Work out the finished part from the listing and answer in its coordinate system (mm). Coordinates: 2 decimals unless noted, no trailing zeros. Loops run counter-clockwise (first coordinate to the right, second up) from the corner with the lowest first, then second, coordinate; pieces in that order, holes last. Notation, with made-up numbers: (80.5, -39) - (128.5, -39) arc R29 ccw to (128.5, -11) - close; hole circle Ø7 at (5.5, 1.5). An arc over 180 degrees is marked (long way). Write each question's results on one line, items separated by ' | '. Start each with the question number.
Item 1: For a pull along Y with two mould halves and no side action, classify faces 1 (the face through (-80.22, -125.83, -2.13)), 2 (the face through (-101, 112, 152.4)), 3 (the face through (19.839, -151.103, 2.134)) as +Y half, -Y half, draft (parallel to the pull), parting line (faces both ways), or undercut.
Item 2: Section B-B, the plane x = 93 is taken. Write down the section's boundary in (y, z).
Item 3: Section A-A, the plane y = 0 is taken. Write down the section's boundary in (x, z) (3 decimals).
Item 4: Section C-C, the plane z = 51.5 is taken. Write down the section's boundary in (x, y) (3 decimals).
Item 5: Consider probe 1 along Y at (x, z) = (0, 75) (3 decimals); probe 2 along Y at (x, z) = (0, -57) (3 decimals); probe 3 along X at (y, z) = (-79, 74.5). Determine where each line is inside the solid, lowest interval first. Write a range as [from, to].
Item 6: Section D-D, the plane x = 0 is taken. Count the separate pieces of the cut face and the enclosed holes in it, plus the area to 3 significant figures.
Item 7: Each of these flat-tipped pins is pushed along its axis until it touches: pin 1 Ø1.5 at (x, z) = (25.5, -77) entering from +Y; pin 2 Ø2 at (y, z) = (44.5, -21) entering from +X; pin 3 Ø12 at (x, z) = (-88.5, 27) entering from +Y. Where does it stop, or does it pass through?
from build123d import *

# Parameters (mm, degrees)
SKETCH3_R                                = 152.4
SKETCH3_R_2                              = 149.225
BOSS_EXTRUDE1_DEPTH                      = 152.4
F_1_0MM_DOWEL_HOLE1_REACH                = 394.408
F_1_0MM_DOWEL_HOLE1_BORE_R               = 38.5
F_1_2_0_5_DIAMETER_HOLE1_REACH           = 394.606
F_1_2_0_5_DIAMETER_HOLE1_BORE_R          = 6.35
F_1_2_0_5_DIAMETER_HOLE1_ON_FACE_2_REACH = 387.1
F_1_2_0_5_DIAMETER_HOLE1_BORE_2_R        = 6.35


with BuildPart() as part:
    # Sketch3 → Boss-Extrude1 (new, symmetric)
    with BuildSketch(Plane.XY):
        with Locations(Location((0, 0, 0), (0, 0, 180))):
            Circle(SKETCH3_R)
        with Locations(Location((0, 0, 0), (0, 0, 180))):
            Circle(SKETCH3_R_2, mode=Mode.SUBTRACT)
    extrude(amount=BOSS_EXTRUDE1_DEPTH, both=True)

    # Ø1.0mm Dowel Hole1 bore (on position points) → Ø1.0mm Dowel Hole1 (cut, up to next)
    with BuildSketch(Plane(origin=(-1.237560308, 152.394975129, -41.195571985), x_dir=(0.999967028404, 0.008120474463, 0), z_dir=(-0.008120474463, 0.999967028404, 0)), mode=Mode.PRIVATE) as f_1_0mm_dowel_hole1_sk1:
        Circle(F_1_0MM_DOWEL_HOLE1_BORE_R)
    f_1_0mm_dowel_hole1_tool1 = extrude(f_1_0mm_dowel_hole1_sk1.sketch, amount=-F_1_0MM_DOWEL_HOLE1_REACH, mode=Mode.PRIVATE) & part.part
    add(f_1_0mm_dowel_hole1_tool1.solids().sort_by_distance((-1.23756, 152.394975, -41.195572))[0], mode=Mode.SUBTRACT)

    # 1/2 (0.5) Diameter Hole1 bore (on position points) → 1/2 (0.5) Diameter Hole1 (cut, up to next)
    with BuildSketch(Plane(origin=(-0.547224497, -152.399017534, -42.136286286), x_dir=(-0.999993553373, 0.003590711924, 0), z_dir=(-0.003590711924, -0.999993553373, 0)), mode=Mode.PRIVATE) as f_1_2_0_5_diameter_hole1_sk1:
        Circle(F_1_2_0_5_DIAMETER_HOLE1_BORE_R)
    f_1_2_0_5_diameter_hole1_tool1 = extrude(f_1_2_0_5_diameter_hole1_sk1.sketch, amount=-F_1_2_0_5_DIAMETER_HOLE1_REACH, mode=Mode.PRIVATE) & part.part
    add(f_1_2_0_5_diameter_hole1_tool1.solids().sort_by_distance((-0.547224, -152.399018, -42.136286))[0], mode=Mode.SUBTRACT)

    # 1/2 (0.5) Diameter Hole1 bore 2 (on position points) → 1/2 (0.5) Diameter Hole1 on face 2 (cut, up to next)
    with BuildSketch(Plane(origin=(0.182408166, -152.399890837, 26.814000364), x_dir=(-0.999999283595, -0.001197000339, 0), z_dir=(0.001197000339, -0.999999283595, 0)), mode=Mode.PRIVATE) as f_1_2_0_5_diameter_hole1_on_face_2_sk1:
        Circle(F_1_2_0_5_DIAMETER_HOLE1_BORE_2_R)
    f_1_2_0_5_diameter_hole1_on_face_2_tool1 = extrude(f_1_2_0_5_diameter_hole1_on_face_2_sk1.sketch, amount=-F_1_2_0_5_DIAMETER_HOLE1_ON_FACE_2_REACH, mode=Mode.PRIVATE) & part.part
    add(f_1_2_0_5_diameter_hole1_on_face_2_tool1.solids().sort_by_distance((0.182408, -152.399891, 26.814))[0], mode=Mode.SUBTRACT)


solid = part.part
Answer key:
1) face 1: undercut | face 2: draft | face 3: parting line
2) outline: (-120.73, -152.4) - (-116.7, -152.4) - (-116.7, 152.4) - (-120.73, 152.4) - close; (116.7, -152.4) - (120.73, -152.4) - (120.73, 152.4) - (116.7, 152.4) - close
3) outline: (-152.4, -152.4) - (-149.225, -152.4) - (-149.225, 152.4) - (-152.4, 152.4) - close; (149.225, -152.4) - (152.4, -152.4) - (152.4, 152.4) - (149.225, 152.4) - close
4) outline: circle Ø304.8 at (0, 0); hole circle Ø298.45 at (0, 0)
5) probe 1: y = [-152.4, -149.225], [149.225, 152.4] | probe 2: y = [-152.4, -149.225] | probe 3: x = [-130.33, -126.6], [126.6, 130.33]
6) separate pieces: 5 | enclosed holes: 0 | area: 1,610 mm^2
7) pin 1: stops at y = 150.38 | pin 2: stops at x = 146.06 | pin 3: stops at y = 128.14
